Print and shaded views of the part. All mm, measured from the part's lowest x, y and z. Coordinates: 2 decimals unless noted, no trailing zeros. Order: outer loops, then holes, each group sorted by start corner. A loop starts at its lowest first (then second) coordinate and runs counter-clockwise, first axis right, second up. Notation, with made-up numbers: M 31.5,69 L 67.5,69 A29 cw 67.5,99 Z; hole C 59,34 d10. An arc over 180 degrees is marked long. Return JSON: item names as keys, results as strings.
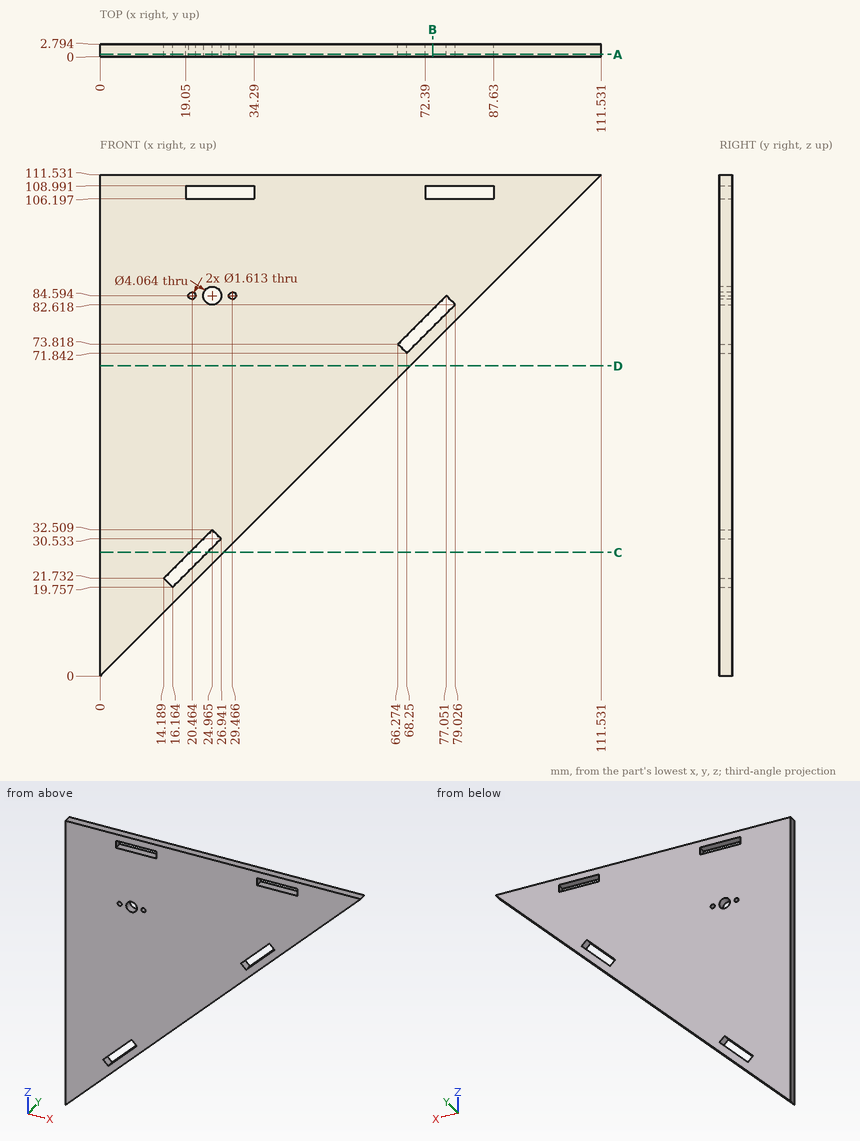
Item 1: Saw through at D-D (z = 69). Write the cut outline in (x, y), and give its area (3 significant figures).
Check result:
{"outline": "M 0,0 L 69,0 L 69,2.79 L 0,2.79 Z", "area": "193 mm2"}
Item 2: Saw through at B-B (x = 74). Write the cut outline in (y, z).
Check result:
{"outline": "M 0,74 L 2.79,74 L 2.79,77.59 L 0,77.59 Z; M 0,81.54 L 2.79,81.54 L 2.79,106.2 L 0,106.2 Z; M 0,108.99 L 2.79,108.99 L 2.79,111.53 L 0,111.53 Z"}
Item 3: Saw through at A-A (y = 0.5). Count the separate pieces of the cut face and the enclosed holes in it, and give its area (3 significant figures).
Check result:
{"separate pieces": "1", "enclosed holes": "7", "area": "6,030 mm2"}
Item 4: Drop flat-ended pins along their axis: pin 1 Ø1.9 at (x, z) = (20.46, 84.59) entering from +Y; pin 2 Ø1.4 at (x, y) = (82.5, 1) entering from -Z; pin 3 Ø3.5 at (x, z) = (24.97, 84.59) entering from +Y (3 decimals); pin 4 Ø0.8 at (y, z) = (1, 108) entering from +X. Give the stop position or say it passes through.
Check result:
{"pin 1": "stops at y = 2.79", "pin 2": "stops at z = 81.8", "pin 3": "passes through", "pin 4": "stops at x = 108.4"}
Item 5: Wall check: line 1 (Z direction, x = 69.5, y = 0.65) (1 decimal); line 2 (X direction, y = 2.7, z = 76) (1 decimal); line 3 (Z direction, x = 21.5, y = 0.35) (1 decimal). Give the ranges that are in metal, low to high.
Check result:
{"line 1": "z = 69.5 to 73.1, 77 to 111.5", "line 2": "x = 0 to 68.5, 72.4 to 76", "line 3": "z = 21.5 to 25.1, 29 to 106.2, 109 to 111.5"}
Item 6: Saw through at C-C (z = 27.5). Write the cut outline in (x, y).
Check result:
{"outline": "M 0,0 L 19.96,0 L 19.96,2.79 L 0,2.79 Z; M 23.91,0 L 27.5,0 L 27.5,2.79 L 23.91,2.79 Z"}
